Verification items for this drawing (mm, ordinates from the low corner). Give positions to 0.01 mm unless a question says otherwise; leave off trailing zeros. Loops run counter-clockwise (first coordinate to the right, second up) from the corner with the lowest first, then second, coordinate; pieces in that order, holes last. Notation, with made-up numbers: M 70.5,-4.5 L 95.5,-4.5 A12 cw 95.5,12.5 Z; hole C 75.5,-6 d2. An arc over 180 degrees is marked long. Put each result on its own line as item: value. Start each with the question number.
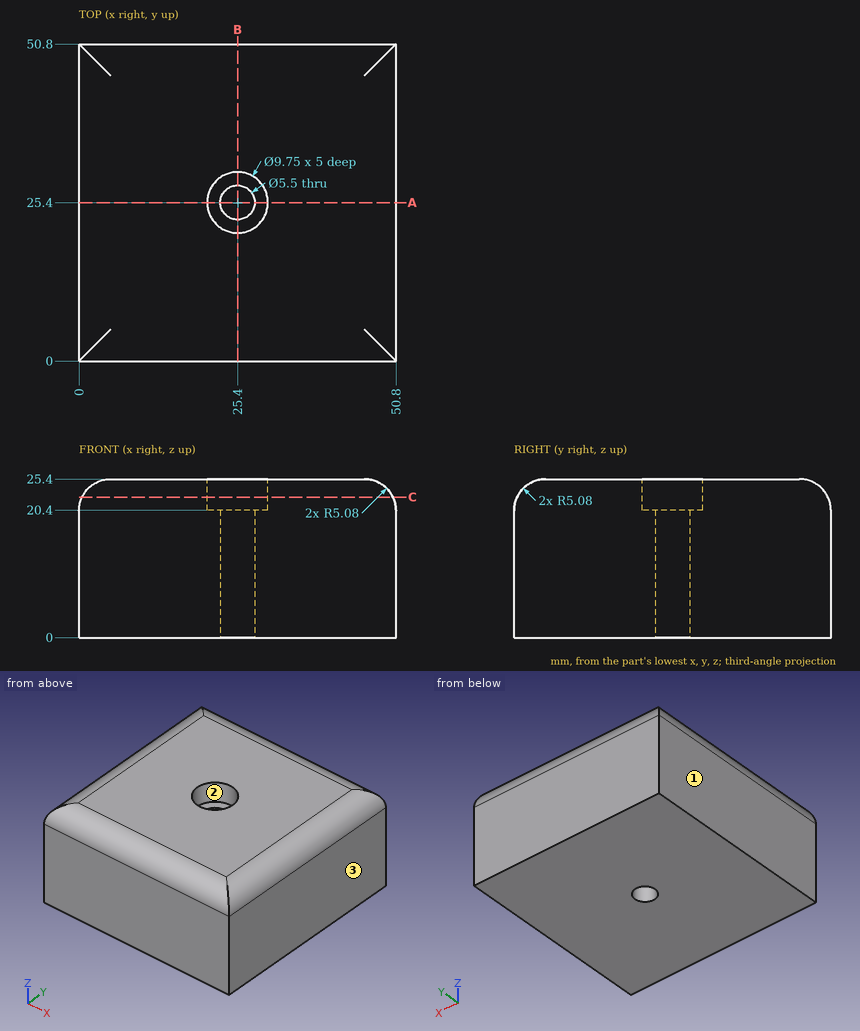
Q1. Cross-section at A-A, the plane y = 25.4. Record the boundary of the cut face in (x, z) (3 decimals).
Q2. Release check for a two-part mould opening along X. For the marked faces 1, 2 and 3 record: pulls with the +X half, pulls with the -X half, needs draft (parallel to the pull), parting line crosses it, or undercut.
Q3. Cross-section at C-C, the plane z = 22.5. Record the boundary of the cut face in (x, y) (3 decimals), then the cut area to 3 significant figures.
Q4. Go/stop test with flat-tipped pins: pin 1 (3 mm diameter, centred on y = 5.5, z = 11.5, fed in from -X); pin 2 (1 mm diameter, centred on x = 27, y = 23.5, fed in from +Z); pin 3 (3.5 mm diameter, centred on x = 25.4, y = 25.4, fed in from +Z). Record where each tip stops, or that it passes through.
Q5. Scan lines: L1, parallel to Y at x = 25.4, z = 16.25; L2, parallel to X at y = 25, z = 1.75; L3, parallel to Y at x = 25.4, z = 24.25 (3 decimals). Record each from-to range of solid material in increasing order.
Ans:
1. outline: M 0,0 L 22.65,0 L 22.65,20.4 L 20.525,20.4 L 20.525,25.4 L 5.08,25.4 A5.08 ccw 0,20.32 Z; M 28.15,0 L 50.8,0 L 50.8,20.32 A5.08 ccw 45.72,25.4 L 30.275,25.4 L 30.275,20.4 L 28.15,20.4 Z
2. face 1: pulls with the -X half
2. face 2: undercut
2. face 3: pulls with the +X half
3. outline: M 0.492,0.492 L 50.308,0.492 L 50.308,50.308 L 0.492,50.308 Z; hole C 25.4,25.4 d9.75
3. area: 2,410 mm^2
4. pin 1: stops at x = 0
4. pin 2: stops at z = 20.4
4. pin 3: passes through
5. L1: y = 0 to 22.65, 28.15 to 50.8
5. L2: x = 0 to 22.68, 28.12 to 50.8
5. L3: y = 1.861 to 20.525, 30.275 to 48.939
